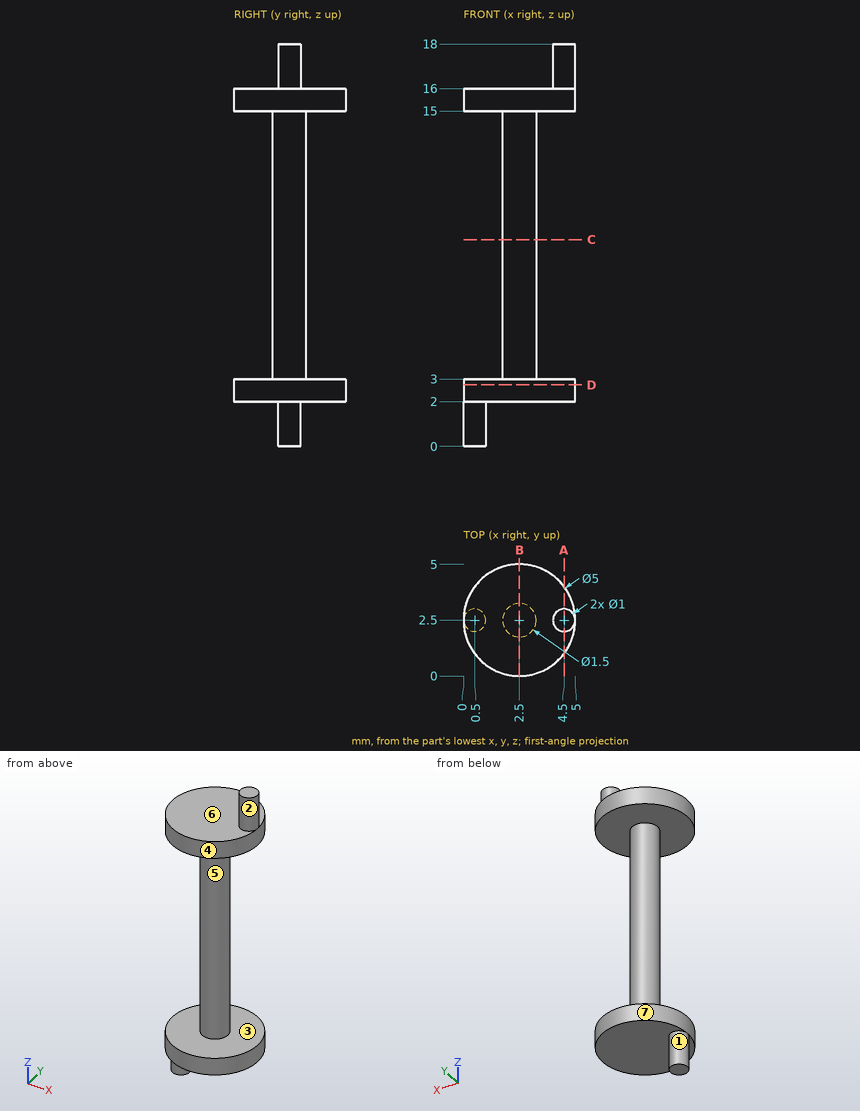
Here's the drawing with two shaded views (mm, measured from the low corner). I have some questions. A direction names the side the tool comes from. Coordinates: 2 decimals unless noted, no trailing zeros. Write each loop counter-clockwise with the first axis right and the second up, starting at its lowest first coordinate (ties: lowest second). Pieces come first, ordered by that corner, then holes. Notation, with made-up numbers: (33, 38.5) -> (63, 38.5) arc R10 cw to (63, 53.5) -> close; hole circle Ø6 at (33, 16). An arc over 180 degrees is marked (long way). One line per question, with ' | ' between items. Start each with the question number.
1. Please list where these lines run through material, in increasing order: line 1 along Z through (x, y) = (3.7, 2.3); line 2 along Z through (x, y) = (1.9, 2.2); line 3 along Y through (x, z) = (2, 11).
2. If we section it at C-C (z = 9.25): Please give me the cut outline in (x, y), and give its area (3 significant figures).
3. If we section it at B-B (x = 2.5): Please give me the cut outline in (y, z), and give its area (3 significant figures).
4. Thinking about a two-plate mould opening in Z: for the marked faces 5, 6 and 7, which applies, pulls with the +Z half, pulls with the -Z half, needs draft (parallel to the pull), parting line crosses it, or undercut?
5. For the marked faces 1, 2, 3 and 4, which set-ups out of +Z, -Z, +X, -X, +Y, -Y let a thin tool reach every point of the face, with its end or its side?
6. If we section it at D-D (z = 2.75): Please give me the cut outline in (x, y).
7. Will these pins go through, and if not, where does the flat tip stop? P1, Ø2, axis at x = 2, y = 3, coming from the -Z side; P2, Ø1.5, axis at x = 3, y = 1.5, coming from the +Z side.
8. If we section it at A-A (x = 4.5): Please give me the cut outline in (y, z), and give its area (3 significant figures).
Return value:
1) line 1: z = 2 to 3, 15 to 16 | line 2: z = 2 to 16 | line 3: y = 1.94 to 3.06
2) outline: circle Ø1.5 at (2.5, 2.5) | area: 1.77 mm²
3) outline: (0, 2) -> (5, 2) -> (5, 3) -> (3.25, 3) -> (3.25, 15) -> (5, 15) -> (5, 16) -> (0, 16) -> (0, 15) -> (1.75, 15) -> (1.75, 3) -> (0, 3) -> close | area: 28.0 mm²
4) face 5: undercut | face 6: pulls with the +Z half | face 7: needs draft
5) face 1: -Z | face 2: +Z | face 3: none | face 4: +Z, -Z
6) outline: circle Ø5 at (2.5, 2.5)
7) P1: stops at z = 2 | P2: stops at z = 16
8) outline: (1, 2) -> (4, 2) -> (4, 3) -> (1, 3) -> close; (1, 15) -> (4, 15) -> (4, 16) -> (3, 16) -> (3, 18) -> (2, 18) -> (2, 16) -> (1, 16) -> close | area: 8.00 mm²
